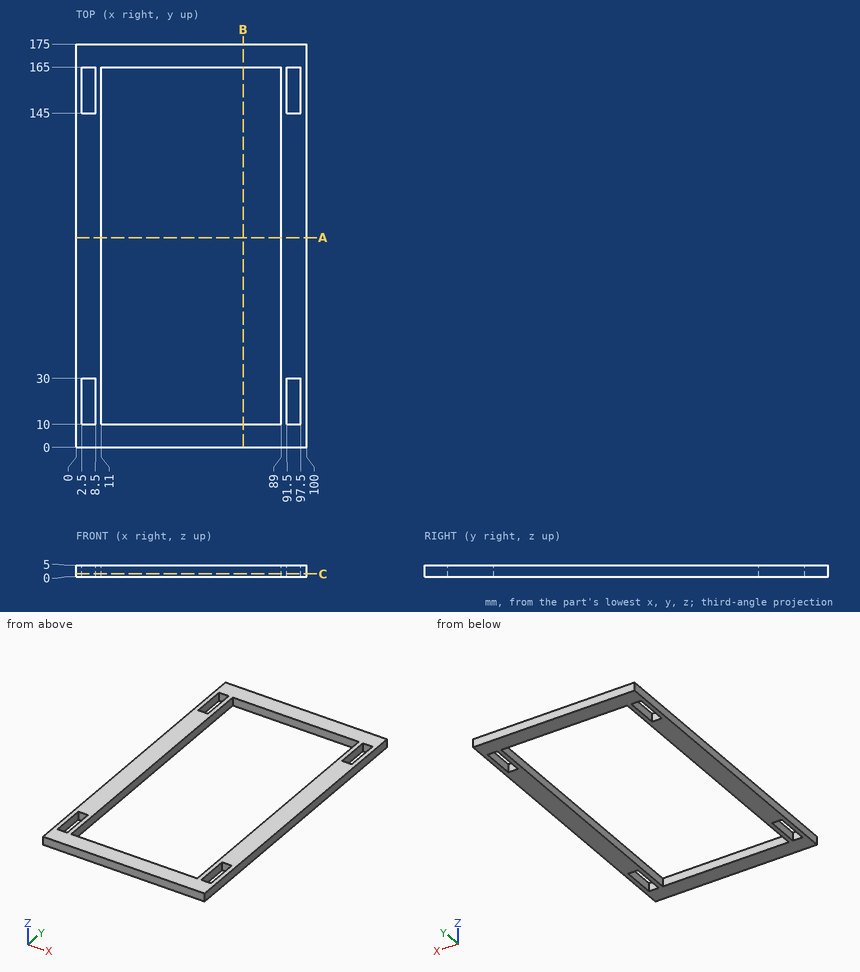
Study the drawing (mm; zero at the part's minimum x, y, z) and answer. Round coordinates to 2 decimals unless told otherwise and drop trailing zeros. Loops run counter-clockwise (first coordinate to the right, second up) from the corner with the lowest first, then second, coordinate; pieces in that order, holes last. Notation, with made-up numbers: (52.5, -12) -> (106.5, -12) arc R29 ccw to (106.5, 26) -> close; hole circle Ø2 at (53.25, 56). An arc over 180 degrees is marked (long way). Use one line per item in the form item = value.
1. The part is cut by section B-B on x = 72.5. Determine the outline of the cut face in (y, z), and give its area (3 significant figures).
Answer key:
outline = (0, 0) -> (10, 0) -> (10, 5) -> (0, 5) -> close; (165, 0) -> (175, 0) -> (175, 5) -> (165, 5) -> close
area = 100 mm²
2. Find the intervals of material crossed by probe 1 along X at (y, z) = (164, 1.55); probe 2 along Y at (x, z) = (14, 4.8); probe 3 along X at (y, z) = (101, 1.7), in increasing order. Write a range as [from, to].
Answer key:
probe_1 = [0, 2.5], [8.5, 11], [89, 91.5], [97.5, 100]
probe_2 = [0, 10], [165, 175]
probe_3 = [0, 11], [89, 100]
3. The part is cut by section C-C on z = 1.4. Determine the outline of the cut face in (x, y), and give its area (3 significant figures).
Answer key:
outline = (0, 0) -> (100, 0) -> (100, 175) -> (0, 175) -> close; hole (2.5, 10) -> (8.5, 10) -> (8.5, 30) -> (2.5, 30) -> close; hole (2.5, 145) -> (8.5, 145) -> (8.5, 165) -> (2.5, 165) -> close; hole (11, 10) -> (89, 10) -> (89, 165) -> (11, 165) -> close; hole (91.5, 10) -> (97.5, 10) -> (97.5, 30) -> (91.5, 30) -> close; hole (91.5, 145) -> (97.5, 145) -> (97.5, 165) -> (91.5, 165) -> close
area = 4,930 mm²
4. The part is cut by section A-A on y = 91. Determine the outline of the cut face in (x, z), and give its area (3 significant figures).
Answer key:
outline = (0, 0) -> (11, 0) -> (11, 5) -> (0, 5) -> close; (89, 0) -> (100, 0) -> (100, 5) -> (89, 5) -> close
area = 110 mm²
